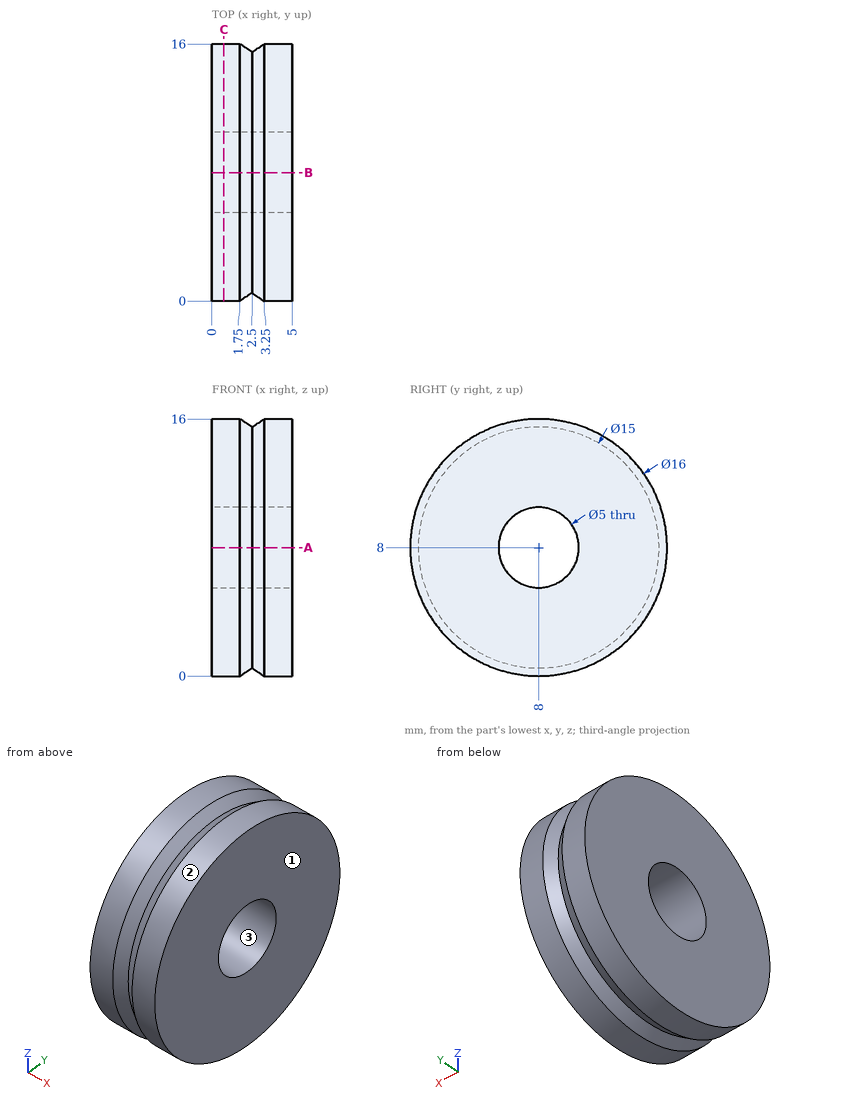
Job drawing, mm, ordinate dimensions from the low corner. One solid piece. Coordinates: 2 decimals unless noted, no trailing zeros. Write each loop counter-clockwise with the first axis right and the second up, starting at its lowest first coordinate (ties: lowest second). Pieces come first, ordered by that corner, then holes. Notation, with made-up numbers: (10, 9) -> (54, 9) arc R22 cw to (54, 20) -> close; hole circle Ø9 at (-19.75, 21). An arc over 180 degrees is marked (long way). Use CSV: the item, a comma, the result in double quotes. Start each with the question number.
Item 1: Band-saw the part on C-C, the plane x = 0.75. Write the cut outline in (y, z), plus the area to 3 significant figures.
Item 2: Band-saw the part on A-A, the plane z = 8. Write the cut outline in (x, y).
Item 3: Wall check: probe 1 along Y at (x, z) = (1.1, 8); probe 2 along Y at (x, z) = (3.1, 8); probe 3 along Z at (x, y) = (3.7, 5.75). Give the ranges that are in metal, low to high.
Item 4: Two-plate mould, pull along Y, no slides. Class the marked faces 1, 2 and 3: +Y half, -Y half, draft (parallel to the pull), parting line (faces both ways), or undercut.
Item 5: Drop flat-ended pins along their axis: P1, Ø2, axis at x = 2, z = 6, coming from the -Y side; P2, Ø1.5, axis at x = 2, y = 10, coming from the +Z side; P3, Ø2, axis at x = 1.5, z = 2, coming from the -Y side (3 decimals). Give the stop position or say it passes through.
Response values:
1,outline,"circle Ø16 at (8, 8); hole circle Ø5 at (8, 8)"
1,area,"181 mm2"
2,outline,"(0, 0) -> (1.75, 0) -> (2.5, 0.5) -> (3.25, 0) -> (5, 0) -> (5, 5.5) -> (0, 5.5) -> close; (0, 10.5) -> (5, 10.5) -> (5, 16) -> (3.25, 16) -> (2.5, 15.5) -> (1.75, 16) -> (0, 16) -> close"
3,probe 1,"y = 0 to 5.5, 10.5 to 16"
3,probe 2,"y = 0.1 to 5.5, 10.5 to 15.9"
3,probe 3,"z = 0.32 to 6.91, 9.09 to 15.68"
4,face 1,"draft"
4,face 2,"parting line"
4,face 3,"undercut"
5,P1,"stops at y = 0.07"
5,P2,"stops at z = 15.89"
5,P3,"stops at y = 1.755"
